Job drawing, mm, ordinate dimensions from the low corner. One solid piece. Give positions to 0.01 mm unless a question says otherwise; leave off trailing zeros. Loops run counter-clockwise (first coordinate to the right, second up) from the corner with the lowest first, then second, coordinate; pieces in that order, holes last. Notation, with made-up numbers: (59, 50) -> (85, 50) arc R18 cw to (85, 62) -> close; hole circle Ø4 at (-26.75, 55). An arc over 180 degrees is marked (long way). Use one line per item in the form item = value.
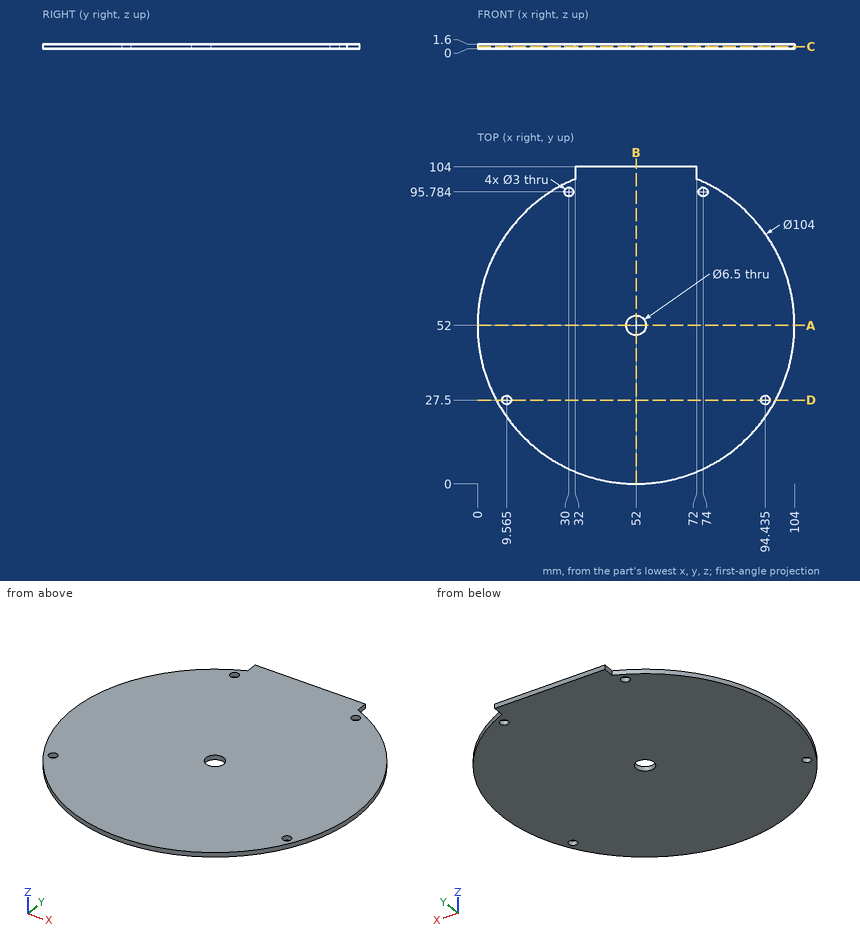
1. Drill centre lines: line 1 (Y direction, x = 52, z = 1.15); line 2 (X direction, y = 50, z = 0.85); line 3 (X direction, y = 94.5, z = 1.3) (1 decimal). Where is each one in solid material? Low to high.
Result sheet:
line_1 = 0 to 48.75, 55.25 to 104
line_2 = 0.04 to 49.44, 54.56 to 103.96
line_3 = 22 to 29.2, 30.8 to 73.2, 74.8 to 82
2. Cut at A-A, the plane y = 52. Write the cut outline in (x, z), then the cut area to 3 significant figures.
Result sheet:
outline = (0, 0) -> (48.75, 0) -> (48.75, 1.6) -> (0, 1.6) -> close; (55.25, 0) -> (104, 0) -> (104, 1.6) -> (55.25, 1.6) -> close
area = 156 mm^2
3. Cut at D-D, the plane y = 27.5. Write the cut outline in (x, z) (1 decimal), then the cut area to 3 significant figures.
Result sheet:
outline = (6.1, 0) -> (8.1, 0) -> (8.1, 1.6) -> (6.1, 1.6) -> close; (11.1, 0) -> (92.9, 0) -> (92.9, 1.6) -> (11.1, 1.6) -> close; (95.9, 0) -> (97.9, 0) -> (97.9, 1.6) -> (95.9, 1.6) -> close
area = 137 mm^2
4. Drop flat-ended pins along their axis: P1, Ø0.8, axis at y = 102, z = 0.5, coming from the -X side; P2, Ø0.8, axis at y = 102, z = 1, coming from the +X side. Give the stop position or say it passes through.
Result sheet:
P1 = 32
P2 = 72
5. Cut at C-C, the plane z = 0.75. State how many separate pieces and enclosed holes the cut face has, then the cut area to 3 significant figures.
Result sheet:
separate_pieces = 1
enclosed_holes = 5
area = 8,490 mm^2
